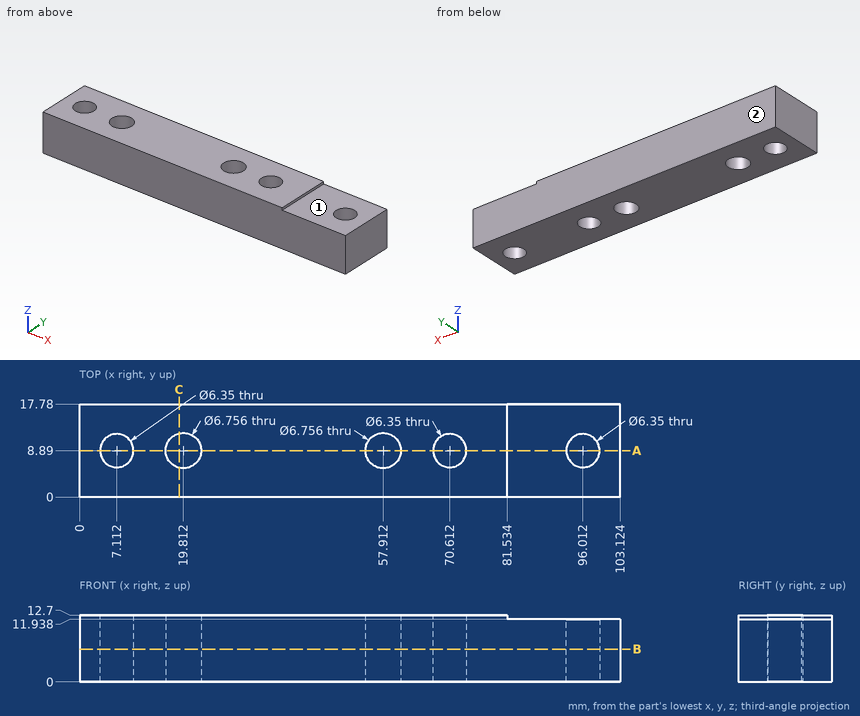
The drawing under review shows one solid part. Ordinate dimensions are in mm from its lowest x, y, z. A direction names the side the tool comes from. Coordinates: 2 decimals unless noted, no trailing zeros. Order: outer loops, then holes, each group sorted by start corner. A loop starts at its lowest first (then second) coordinate and runs counter-clockwise, first axis right, second up. Notation, with made-up numbers: (6.5, 55) - (32.5, 55) arc R32 ccw to (32.5, 91) - close; hole circle Ø9 at (-10, -34.5). An arc over 180 degrees is marked (long way). Put each result on its own line as item: value.
1) Insertion check: P1, Ø5, axis at x = 96.012, y = 8.89, coming from the +Z side; P2, Ø9, axis at x = 96.5, y = 11.5, coming from the +Z side. Each pin has a flat end and moves straight along its axis. Give the tip position at first contact, or say it passes through.
Response values:
P1: passes through
P2: stops at z = 11.94
2) Wall thickness on L1, parallel to X at y = 6, z = 10 (1 decimal); L2, parallel to Y at x = 20, z = 8.5; L3, parallel to Z at x = 90, y = 7.25: over which ranges is each line inside the solid? List them lowest first. Write a range as from..to.
Response values:
L1: x = 0..5.8, 8.4..18.1, 21.6..56.2, 59.7..69.3, 71.9..94.7, 97.3..103.1
L2: y = 0..5.52, 12.26..17.78
L3: z = 0..11.94
3) Take a section at B-B, the plane z = 6.25. Count the separate pieces of the cut face and the enclosed holes in it, and give its area (3 significant figures).
Response values:
separate pieces: 1
enclosed holes: 5
area: 1,670 mm²
4) Tool access review of the marked faces 1 and 2: name each direction out of +Z, -Z, +X, -X, +Y, -Y from which nothing blocks a thin tool from reaching the whole face with its end or side.
Response values:
face 1: +Z, +X, +Y, -Y
face 2: +Z, -Z, +X, -X, +Y
5) Take a section at A-A, the plane y = 8.89. Give the boundary of the cut face in (x, z).
Response values:
outline: (0, 0) - (3.94, 0) - (3.94, 12.7) - (0, 12.7) - close; (10.29, 0) - (16.43, 0) - (16.43, 12.7) - (10.29, 12.7) - close; (23.19, 0) - (54.53, 0) - (54.53, 12.7) - (23.19, 12.7) - close; (61.29, 0) - (67.44, 0) - (67.44, 12.7) - (61.29, 12.7) - close; (73.79, 0) - (92.84, 0) - (92.84, 11.94) - (81.53, 11.94) - (81.53, 12.7) - (73.79, 12.7) - close; (99.19, 0) - (103.12, 0) - (103.12, 11.94) - (99.19, 11.94) - close
6) Take a section at C-C, the plane x = 19. Give the boundary of the cut face in (y, z).
Response values:
outline: (0, 0) - (5.61, 0) - (5.61, 12.7) - (0, 12.7) - close; (12.17, 0) - (17.78, 0) - (17.78, 12.7) - (12.17, 12.7) - close
